Could you check a few things on this model? Use its own coordinates, in mm. A direction names the side the tool comes from. Round coordinates to 2 decimals unless told otherwise and drop trailing zeros. Loops run counter-clockwise (first coordinate to the right, second up) from the corner with the lowest first, then second, coordinate; pieces in that order, holes last. Notation, with made-up numbers: (11.25, -3) - (45.25, -3) arc R34 cw to (45.25, 30) - close; hole circle Ø2 at (-5.75, 38). An arc over 180 degrees is marked (long way). Answer as CSV lines item,"result". Start each with the question number.
1) Suppose I cut it at D-D, the plane z = -15.75. Write out the boundary of the cut face in (x, y) (3 decimals).
2) Please list where these lines run through material, in increasing order: line 1 along X through (y, z) = (-9, -7) (3 decimals); line 2 along X through (y, z) = (-6.5, -2); line 3 along X through (y, z) = (-6.25, -18).
3) Which directions (+Z, -Z, +X, -X, +Y, -Y) give clear straight access to the entire face, cutting with the end or side of a thin tool? Please do faces 4 (the face through (-15, -6.35, -14)), 5 (the face through (-11, -7.6, -13)), 6 (the face through (11, -6, -21.7)).
4) I'm going to push flat-ended pins straight in: pin 1 Ø3 at (y, z) = (-4, -9.5) entering from -X; pin 2 Ø2.5 at (x, z) = (-4, -20) entering from +Y; pin 3 Ø0.6 at (y, z) = (-6.5, -27) entering from +X; pin 4 Ø3.5 at (x, z) = (-15.375, -7) entering from -Y. Where does each tip first touch, or does it pass through?
5) Suppose I cut it at B-B, the plane y = -8. Write out the boundary of the cut face in (x, z) (3 decimals).
6) We'd pull the mould along X, two halves only. Please class faces 1 (the face through (-2, -3, -14)), 2 (the face through (-11, -7.05, -27)), 3 (the face through (-6, -6.35, -14)): pulls with the +X half, pulls with the -X half, needs draft (parallel to the pull), parting line crosses it, or undercut.
7) Suppose I cut it at A-A, the plane z = -7. Write out the boundary of the cut face in (x, y) (3 decimals).
8) Suppose I cut it at C-C, the plane z = -20.7. Write out the boundary of the cut face in (x, y) (3 decimals), then the cut area to 3 significant figures.
Autodesk Inventor part; units mm, degrees
ref_plane "Arbeitsebene1" through (0, 0, -12.7) normal (0, 0, -1) x (-1, 0, 0)
ref_plane "YZ Plane" through (0, 0, 0) normal (1, 0, 0) x (0, 1, 0)
ref_plane "XZ Plane" through (0, 0, 0) normal (0, 1, 0) x (-1, 0, 0)
ref_plane "Arbeitsebene1" through (0, 0, -12.7) normal (0, 0, -1) x (-1, 0, 0)
sketch "Skizze2" plane through (0, 0, -12.7) normal (0, 0, -1) x (-1, 0, 0)
  line L0 (-55.25, 0) -> (-55.25, -12.7)
  line L1 (0, -12.7) -> (-55.25, -12.7)
  line L2 (0, 0) -> (0, -12.7)
  line L3 (0, 0) -> (-55.25, 0)
  circle A0 centre (-47.625, -6.35) radius 2.75
  circle A1 centre (-7.625, -6.35) radius 2.75
  line L4 (0, 1.15) -> (-15, 1.15)
  line L5 (-15, 1.15) -> (-15, -13.85)
  line L6 (-15, -13.85) -> (0, -13.85)
  line L7 (0, -13.85) -> (0, 1.15)
  point P0 (-15, -6.35)
  dimension "d1" = 15
  dimension "d2" = 0
  dimension "d3" = 15
extrude "Extrusion1" add sketch "Skizze2" along normal blind 15 contours L5 L4 L7 L3 | L3 L2 L1 L5 | L1 L7 L6 L5 | A1
sketch "Skizze3" plane through (0, -13.85, -12.7) normal (-1, 0, 0) x (0, 0, 1)
  line L0 (12.7, 1.15) -> (12.7, 13.85)
  line L1 (-15, 0) -> (-15, 15)
  line L2 (-15, 15) -> (12.7, 15)
  line L3 (12.7, 15) -> (12.7, 0)
  line L4 (12.7, 0) -> (-15, 0)
  line L5 (-15, 0) -> (-15, 15)
  line L6 (0, 0) -> (-15, 0)
extrude "Extrusion2" add sketch "Skizze3" along normal blind 2
sketch "Skizze4" plane through (-2, -13.85, -12.7) normal (-1, 0, 0) x (0, 0, 1)
  line L0 (0, 0) -> (12.7, 0)
  line L1 (-15, 15) -> (-15, 0)
  line L2 (12.7, 0) -> (-15, 0)
  line L3 (-15, 0) -> (-15, 7.5)
  line L4 (-15, 7.5) -> (12.7, 7.5)
  line L5 (12.7, 7.5) -> (12.7, 0)
  line L6 (12.7, 0) -> (12.7, 15)
  point P0 (12.7, 13.85)
  point P1 (12.7, 7.5)
  point P2 (-1.15, 7.5)
extrude "Extrusion3" add sketch "Skizze4" along normal blind 17
sketch "Skizze5" plane through (-2, -6.35, 0) normal (0, 1, 0) x (1, 0, 0)
  line L0 (0, 27.7) -> (-17, 27.7)
  line L1 (0, 0) -> (0, 27.7)
  line L2 (0, 0) -> (-17, 0)
  line L3 (-17, 0) -> (-17, 27.7)
  line L4 (-7.25, 0) -> (-9.75, 0)
  line L5 (-9.75, 0) -> (-9.75, 25.75)
  line L6 (-9.75, 25.75) -> (-7.25, 25.75)
  line L7 (-7.25, 25.75) -> (-7.25, 0)
  point P0 (2, 0)
  point P1 (-8.5, 0)
  point P2 (-8.5, 0)
  dimension "d10" = 2.5
  dimension "d17" = 25.75
extrude "Extrusion4" cut sketch "Skizze5" against normal blind 1.25 contours L2 L5 L6 L7
sketch "Skizze6" plane through (-2, -6.35, 0) normal (0, 1, 0) x (1, 0, 0)
  line L0 (-9.75, 25.75) -> (-7.25, 25.75)
  line L1 (-7.25, 25.75) -> (-7.25, 0)
  line L2 (-9.75, 0) -> (-9.75, 25.75)
  line L3 (0, 27.7) -> (-17, 27.7)
  line L4 (-9.75, 25.75) -> (-7.25, 25.75)
  line L5 (-7.8, 25.75) -> (-9.2, 25.75)
  line L6 (-9.2, 25.75) -> (-9.2, 27.7)
  line L7 (-9.2, 27.7) -> (-7.8, 27.7)
  line L8 (-7.8, 27.7) -> (-7.8, 25.75)
  point P0 (2, 0)
  point P1 (-8.5, 25.75)
  point P2 (-8.5, 25.75)
  point P3 (-7.8, 27.7)
  dimension "d14" = 1.4
extrude "Extrusion5" cut sketch "Skizze6" against normal blind 0.7
sketch "Skizze7" plane through (-2, -6.35, 0) normal (0, 1, 0) x (1, 0, 0)
  circle A0 centre (-3.625, 7) radius 2
  circle A1 centre (-13.375, 7) radius 2
  circle A2 centre (-13.375, 20.7) radius 2
  circle A3 centre (-3.625, 20.7) radius 2
  line L0 (0, 0) -> (-7.25, 0)
  line L1 (-9.75, 0) -> (-17, 0)
  line L2 (-9.2, 27.7) -> (-17, 27.7)
  point P0 (2, 0)
  point P1 (-3.625, 0)
  point P2 (-13.375, 0)
  dimension "d18" = 4
  dimension "d19" = 4
  dimension "d20" = 4
  dimension "d21" = 4
  dimension "d22" = 7
  dimension "d23" = 7
extrude "Extrusion6" cut sketch "Skizze7" against normal blind 10
sketch "Skizze9" plane through (0, 0, -27.7) normal (0, 0, -1) x (-1, 0, 0)
  circle A0 centre (-7.625, -6.35) radius 2.75
  point P0 (0, 0)
hole "Bohrung1" at (7.625, -6.35, -27.7) direction (0, 0, 1) diameter 5.6 depth 15 counterbore diameter 9 counterbore depth 6
sketch "Skizze10" plane through (0, 1.15, -12.7) normal (0, 1, 0) x (1, 0, 0)
  line L0 (19, -16) -> (-4, -16)
  line L1 (-4, -16) -> (-4, 20)
  line L2 (-4, 20) -> (19, 20)
  line L3 (19, 20) -> (19, -16)
  point P0 (0, -12.7)
extrude "Extrusion8" cut sketch "Skizze10" against normal blind 1.15
sketch "Skizze11" plane through (15, -13.85, -27.7) normal (0, -1, 0) x (1, 0, 0)
  line L0 (6, 49) -> (-39, 49)
  line L1 (-39, 49) -> (-39, -17)
  line L2 (-39, -17) -> (6, -17)
  line L3 (6, -17) -> (6, 49)
  point P0 (-15, 27.7)
extrude "Extrusion9" cut sketch "Skizze11" against normal blind 1.15
fillet "Rundung2" radius 2 5 edges at (-19, -9.525, -27.7) (-19, -9.525, 0) (15, -6.35, -27.7) (15, 0, -20.2) (6.5, 0, -27.7)
equation "\"d19\" = d18"
equation "\"d20\" = d19"
equation "\"d21\" = d19"
equation "\"d23\" = d22"
properties part number "NadelhalterSchraub"
Filled sheet:
1,outline,"(-19, -12.7) - (15, -12.7) - (15, -2) arc R2 ccw to (13, 0) - (-2, 0) - (-2, -6.35) - (-9.25, -6.35) - (-9.25, -7.6) - (-11.75, -7.6) - (-11.75, -6.35) - (-19, -6.35) - close; hole circle Ø5.6 at (7.625, -6.35)"
2,line 1,"-19 to -17.375, -13.375 to -7.625, -3.625 to 0"
2,line 2,"-19 to -11.75, -9.25 to 0"
2,line 3,"-2 to 4.83, 10.42 to 15"
3,face 4,"+Z, -Z, -X, +Y"
3,face 5,"+Z, +Y"
3,face 6,"-Z"
4,pin 1,"x = -2"
4,pin 2,"y = -6.35"
4,pin 3,"x = 14.73"
4,pin 4,"through"
5,outline,"(-19, -25.7) arc R2 ccw to (-17, -27.7) - (3.438, -27.7) - (3.438, -21.7) - (5.363, -21.7) - (5.363, -12.7) - (0, -12.7) - (0, 0) - (-17, 0) arc R2 ccw to (-19, -2) - close; (9.887, -21.7) - (11.812, -21.7) - (11.812, -27.7) - (13, -27.7) arc R2 ccw to (15, -25.7) - (15, -12.7) - (9.887, -12.7) - close; hole circle Ø4 at (-15.375, -20.7); hole circle Ø4 at (-15.375, -7); hole circle Ø4 at (-5.625, -20.7); hole circle Ø4 at (-5.625, -7)"
6,face 1,"pulls with the -X half"
6,face 2,"undercut"
6,face 3,"needs draft"
7,outline,"(-19, -12.7) - (-17.375, -12.7) - (-17.375, -6.35) - (-19, -6.35) - close; (-13.375, -12.7) - (-7.625, -12.7) - (-7.625, -6.35) - (-9.25, -6.35) - (-9.25, -7.6) - (-11.75, -7.6) - (-11.75, -6.35) - (-13.375, -6.35) - close; (-3.625, -12.7) - (0, -12.7) - (0, 0) - (-2, 0) - (-2, -6.35) - (-3.625, -6.35) - close"
8,outline,"(-19, -12.7) - (-17.375, -12.7) - (-17.375, -6.35) - (-19, -6.35) - close; (-13.375, -12.7) - (-7.625, -12.7) - (-7.625, -6.35) - (-9.25, -6.35) - (-9.25, -7.6) - (-11.75, -7.6) - (-11.75, -6.35) - (-13.375, -6.35) - close; (-3.625, -12.7) - (15, -12.7) - (15, -2) arc R2 ccw to (13, 0) - (-2, 0) - (-2, -6.35) - (-3.625, -6.35) - close; hole circle Ø5.6 at (7.625, -6.35)"
8,area,"244 mm²"
